Check sheet for the modelled part. Datum: model origin and axes. Units: mm. A direction names the side the tool comes from. Give positions to 0.01 mm unless a question says otherwise; leave off trailing zeros. Order: outer loops, then holes, each group sorted by start corner. A loop starts at its lowest first (then second) coordinate and runs counter-clockwise, first axis right, second up. Notation, with made-up numbers: (-17.5, -7.75) -> (5.5, -7.75) arc R7 ccw to (5.5, 5.25) -> close; hole circle Ø8 at (41.25, 85). An arc over 180 degrees is marked (long way). One line per question, with ' | ' between items.
```python
from build123d import *

# Parameters (mm, degrees)
BOSS_EXTRUDE1_DEPTH = 60
CUT_EXTRUDE1_DEPTH  = 120
CUT_EXTRUDE2_DEPTH  = 120
CUT_EXTRUDE3_DEPTH  = 60
SKETCH7_R           = 19
CUT_EXTRUDE4_DEPTH  = 60
SKETCH10_R          = 8
SKETCH10_R_2        = 7.507478142
SKETCH10_R_3        = 6
CUT_EXTRUDE5_DEPTH  = 120


with BuildPart() as part:
    # Sketch1 → Boss-Extrude1 (new, symmetric)
    with BuildSketch(Plane.XY):
        Polygon((-112.5, 0), (-112.5, -12), (112.5, -12), (112.5, 0), (42.711972594, 0), (42.711972594, 108), (30.711972594, 108), (30.711972594, 0), (-27.288027406, 0), (-27.288027406, 108), (-39.288027406, 108), (-39.288027406, 0), align=None)
    extrude(amount=BOSS_EXTRUDE1_DEPTH, both=True)

    # Sketch2 → Cut-Extrude1 (cut)
    with BuildSketch(Plane(origin=(0, 0, 0), x_dir=(1, 0, 0), z_dir=(0, 1, 0))):
        Polygon((112.5, -60), (112.5, -40.004428551), (92.5, -60), align=None)
    extrude(amount=-CUT_EXTRUDE1_DEPTH, mode=Mode.SUBTRACT)

    # Sketch3 → Cut-Extrude2 (cut)
    with BuildSketch(Plane(origin=(0, 0, 0), x_dir=(1, 0, 0), z_dir=(0, 1, 0))):
        Polygon((-39.288027406, 60), (-112.5, 60), (-112.5, -21.997416505), align=None)
    extrude(amount=-CUT_EXTRUDE2_DEPTH, mode=Mode.SUBTRACT)

    # Sketch5 → Cut-Extrude3 (cut, symmetric)
    with BuildSketch(Plane(origin=(0, 0, 0), x_dir=(0, 0, -1), z_dir=(1, 0, 0))):
        Polygon((9.388870173, 108), (-60, 108), (-60, 15.855119955), align=None)
    extrude(amount=CUT_EXTRUDE3_DEPTH, both=True, mode=Mode.SUBTRACT)

    # Sketch7 → Cut-Extrude4 (cut, symmetric)
    with BuildSketch(Plane(origin=(0, 0, 0), x_dir=(0, 0, -1), z_dir=(1, 0, 0))):
        with Locations(Location((22, 70, 0), (0, 0, 90))):
            Circle(SKETCH7_R)
    extrude(amount=CUT_EXTRUDE4_DEPTH, both=True, mode=Mode.SUBTRACT)

    # Sketch10 → Cut-Extrude5 (cut)
    with BuildSketch(Plane(origin=(0, 0, 0), x_dir=(1, 0, 0), z_dir=(0, 1, 0))):
        with Locations(Location((0, 39.625914849, 0), (0, 0, 270))):
            Circle(SKETCH10_R)
        with Locations(Location((90, -40, 0), (0, 0, 270))):
            Circle(SKETCH10_R_2)
        with Locations(Location((-92.5, -48, 0), (0, 0, 270))):
            Circle(SKETCH10_R_3)
        with Locations(Location((0, -39.625914849, 0), (0, 0, 180))):
            Circle(SKETCH10_R)
        with Locations(Location((90, 40, 0), (0, 0, 180))):
            Circle(SKETCH10_R_2)
    extrude(amount=-CUT_EXTRUDE5_DEPTH, mode=Mode.SUBTRACT)


solid = part.part
```
Q1. Access from +Z, -Z, +X, -X, +Y, -Y to the whole of each face (thin tool, end or side, straight path). Record for faces 4 (the face through (-4.868, -5.916, -45.974)), 5 (the face through (78, 0, 1)), 6 (the face through (30.712, 43, -12)).
Result sheet:
face 4: +Y, -Y | face 5: +Z, -Z, +X, +Y | face 6: +Z, -Z, +Y
Q2. Section check A-A (z = -35.5). Enter the section's corners in (x, y).
Result sheet:
outline: (-61.16, -12) -> (-6.85, -12) -> (-6.85, 0) -> (-27.29, 0) -> (-27.29, 56.63) -> (-39.29, 56.63) -> (-39.29, 0) -> (-61.16, 0) -> close; (-39.29, 83.37) -> (-27.29, 83.37) -> (-27.29, 108) -> (-39.29, 108) -> close; (6.85, -12) -> (83.99, -12) -> (83.99, 0) -> (42.71, 0) -> (42.71, 56.63) -> (30.71, 56.63) -> (30.71, 0) -> (6.85, 0) -> close; (30.71, 83.37) -> (42.71, 83.37) -> (42.71, 108) -> (30.71, 108) -> close; (96.01, -12) -> (112.5, -12) -> (112.5, 0) -> (96.01, 0) -> close
Q3. Section check D-D (y = 61.5). Enter the section's corners in (x, z).
Result sheet:
outline: (-39.29, -60) -> (-27.29, -60) -> (-27.29, -38.99) -> (-39.29, -38.99) -> close; (-39.29, -5.01) -> (-27.29, -5.01) -> (-27.29, 25.63) -> (-39.29, 25.63) -> close; (30.71, -60) -> (42.71, -60) -> (42.71, -38.99) -> (30.71, -38.99) -> close; (30.71, -5.01) -> (42.71, -5.01) -> (42.71, 25.63) -> (30.71, 25.63) -> close
Q4. Section check C-C (z = -22). Enter the section's corners in (x, y).
Result sheet:
outline: (-73.22, -12) -> (112.5, -12) -> (112.5, 0) -> (42.71, 0) -> (42.71, 51) -> (30.71, 51) -> (30.71, 0) -> (-27.29, 0) -> (-27.29, 51) -> (-39.29, 51) -> (-39.29, 0) -> (-73.22, 0) -> close; (-39.29, 89) -> (-27.29, 89) -> (-27.29, 108) -> (-39.29, 108) -> close; (30.71, 89) -> (42.71, 89) -> (42.71, 108) -> (30.71, 108) -> close
Q5. Mould release check, pull along X, two halves, no side actions. Record for faces 1 (the face through (-112.5, -6, 41)), 2 (the face through (-33.204, 61.283, 25.791)), 3 (the face through (-27.288, 41, -12)): pulls with the +X half, pulls with the -X half, needs draft (parallel to the pull), parting line crosses it, or undercut.
Result sheet:
face 1: pulls with the -X half | face 2: needs draft | face 3: undercut
Q6. Section check B-B (y = 34.5). Enter the section's corners in (x, z), and give its area (3 significant figures).
Result sheet:
outline: (-39.29, -60) -> (-27.29, -60) -> (-27.29, 45.96) -> (-39.29, 45.96) -> close; (30.71, -60) -> (42.71, -60) -> (42.71, 45.96) -> (30.71, 45.96) -> close | area: 2,540 mm2
Q7. Thickness scan on line 1 (X direction, y = 27.5, z = -26); line 2 (Y direction, x = 98.5, z = -29); line 3 (Z direction, x = 42, y = 72). Record the ranges inside material, lowest first.
Result sheet:
line 1: x = -39.29 to -27.29, 30.71 to 42.71 | line 2: y = -12 to 0 | line 3: z = -60 to -40.89, -3.11 to 17.72
Q8. Depth check by flat-ended pin: pin 1 Ø3 at (y, z) = (63.5, -3.5) entering from -X; pin 2 Ø10 at (x, y) = (-3.5, 3) entering from +Z; pin 3 Ø2 at (x, z) = (9, -24) entering from +Y; pin 4 Ø3 at (y, z) = (76, -1.5) entering from +X. Enter the tip coordinate at first touch or a pass-through.
Result sheet:
pin 1: stops at x = -39.29 | pin 2: stops at z = 60 | pin 3: stops at y = 0 | pin 4: stops at x = 42.71
